from build123d import *

# Parameters (mm, degrees)
SKETCH002_R      = 1.8
SKETCH002_W      = 81
SKETCH002_H      = 81
PAD_DEPTH        = 2
SKETCH003_R      = 3.2
POCKET_DEPTH     = 0.8
SKETCH006_R      = 1.8
PAD002_DEPTH     = 0.12
PAD001_DEPTH     = 20
CHAMFER001_SIZE2 = 2.99
CHAMFER001_SIZE  = 7.5
CHAMFER002_SIZE  = 4
FILLET_R         = 4
CHAMFER003_SIZE  = 1
SKETCH005_R      = 2.2
POCKET001_DEPTH  = 33.501
SKETCH010_R      = 2.2
PAD006_DEPTH     = 0.12
SKETCH007_W      = 85
SKETCH007_H      = 85
SKETCH007_W_2    = 81
SKETCH007_H_2    = 81
PAD003_DEPTH     = 7
SKETCH008_W      = 81
SKETCH008_H      = 81
SKETCH008_R      = 2.5
PAD004_DEPTH     = 1.8
CHAMFER_SIZE     = 1.2
SKETCH009_R      = 2.5
PAD005_DEPTH     = 0.12
FILLET001_R      = 2


with BuildPart() as part:
    # Sketch002 → Pad (new body)
    with BuildSketch(Plane.XY):
        with BuildLine():
            Line((-65, 88.5), (-65, 80))
            Line((-65, 80), (-52.5, 67.5))
            Line((-52.5, 67.5), (-52.5, -20))
            Line((-52.5, -20), (-73, -20))
            Line((-73, -20), (-73, -40))
            Line((-73, -40), (-52.5, -40))
            Line((-52.5, -40), (-52.5, -50))
            Line((-52.5, -50), (52.5, -50))
            Line((52.5, -50), (52.5, -40))
            Line((52.5, -40), (91, -40))
            Line((91, -40), (91, -20))
            Line((91, -20), (52.5, -20))
            Line((52.5, -20), (52.5, 67.5))
            Line((52.5, 67.5), (120, 67.5))
            Line((120, 67.5), (133, 80.5))
            Line((133, 80.5), (133, 88.5))
            ThreePointArc((133, 88.5), (131.535534, 92.035534), (128, 93.5))
            Line((128, 93.5), (52.5, 93.5))
            ThreePointArc((52.5, 93.5), (34.115224, 85.884776), (26.5, 67.5))
            Line((26.5, 50), (26.5, 67.5))
            Line((-26.5, 50), (26.5, 50))
            Line((-26.5, 67.5), (-26.5, 50))
            ThreePointArc((-26.5, 67.5), (-34.115224, 85.884776), (-52.5, 93.5))
            Line((-60, 93.5), (-52.5, 93.5))
            ThreePointArc((-60, 93.5), (-63.535534, 92.035534), (-65, 88.5))
        make_face()
        with Locations((-60, 88.5)):
            Circle(SKETCH002_R, mode=Mode.SUBTRACT)
        with Locations((128, 85.5)):
            Circle(SKETCH002_R, mode=Mode.SUBTRACT)
        Rectangle(SKETCH002_W, SKETCH002_H, mode=Mode.SUBTRACT)
    extrude(amount=PAD_DEPTH)

    # Sketch003 → Pocket (cut)
    with BuildSketch(Plane.XY.offset(2)):
        with Locations((-60, 88.5)):
            Circle(SKETCH003_R)
        with Locations((128, 85.5)):
            Circle(SKETCH003_R)
    extrude(amount=-POCKET_DEPTH, mode=Mode.SUBTRACT)

    # Sketch006 → Pad002 (join)
    with BuildSketch(Plane.XY.offset(1.2)):
        with Locations((-60, 88.5)):
            Circle(SKETCH006_R)
        with Locations((128, 85.5)):
            Circle(SKETCH006_R)
    extrude(amount=-PAD002_DEPTH)

    # Sketch004 (on DatumPlane) → Pad001 (join)
    with BuildSketch(Plane(origin=(-87, -40, 0), x_dir=(-1, 0, 0), z_dir=(0, 1, 0))):
        Polygon((-178, 0), (-139.5, 0), (-139.5, -3), (-173, -3), (-173, -33.5), (-192, -33.5), (-192, -28.5), (-178, -28.5), align=None)
        Polygon((-14, 0), (-34.5, 0), (-34.5, -3), (-19, -3), (-19, -33.5), (0, -33.5), (0, -28.5), (-14, -28.5), align=None)
    extrude(amount=PAD001_DEPTH)

    # Chamfer001
    chamfer001_edges = [part.edges().sort_by_distance(p)[0] for p in [
        (-52.5, -30, 0),
        (52.5, -30, 0),
    ]]
    chamfer001_side = part.faces().sort_by_distance((-56.25, 91.054673, 0))[0]
    chamfer(chamfer001_edges, length=CHAMFER001_SIZE, length2=CHAMFER001_SIZE2, reference=chamfer001_side)

    # Chamfer002
    chamfer002_edges = [part.edges().sort_by_distance(p)[0] for p in [
        (91, -30, 2),
        (-73, -30, 2),
    ]]
    chamfer(chamfer002_edges, length=CHAMFER002_SIZE)

    # Fillet
    fillet_edges = [part.edges().sort_by_distance(p)[0] for p in [
        (105, -40, -31),
        (-87, -40, -31),
        (-68, -30, -33.5),
        (86, -30, -33.5),
        (-87, -20, -31),
        (105, -20, -31),
        (86, -30, -3),
        (-68, -30, -3),
        (52.5, -20, 1),
        (52.5, -40, 1),
        (52.5, -50, 1),
        (-52.5, -50, 1),
        (-52.5, -40, 1),
        (-26.5, 50, 1),
        (26.5, 50, 1),
        (52.5, 67.5, 1),
        (120, 67.5, 1),
        (133, 80.5, 1),
        (-52.5, 67.5, 1),
        (-65, 80, 1),
        (-52.5, -20, 1),
    ]]
    fillet(fillet_edges, radius=FILLET_R)

    # Chamfer003
    chamfer003_edges = [part.edges().sort_by_distance(p)[0] for p in [
        (0, 50, 2),
        (0, -50, 2),
        (91, -40, -15.25),
        (89, -40, 0),
        (89, -20, 0),
        (91, -20, -15.25),
        (-71, -40, 0),
        (-71, -20, 0),
        (-73, -20, -15.25),
        (-73, -40, -15.25),
    ]]
    chamfer(chamfer003_edges, length=CHAMFER003_SIZE)

    # Sketch005 → Pocket001 (cut, through all)
    with BuildSketch(Plane.XY):
        with Locations((-80, -30)):
            Circle(SKETCH005_R)
        with Locations((98, -30)):
            Circle(SKETCH005_R)
    extrude(amount=-POCKET001_DEPTH, mode=Mode.SUBTRACT)

    # Sketch010 (on Face105 of Pocket001) → Pad006 (join)
    with BuildSketch(Plane.XY.offset(-28.5)):
        with Locations((-80, -30)):
            Circle(SKETCH010_R)
        with Locations((98, -30)):
            Circle(SKETCH010_R)
    extrude(amount=-PAD006_DEPTH)

    # Sketch007 → Pad003 (join)
    with BuildSketch(Plane.XY):
        Rectangle(SKETCH007_W, SKETCH007_H)
        Rectangle(SKETCH007_W_2, SKETCH007_H_2, mode=Mode.SUBTRACT)
    extrude(amount=-PAD003_DEPTH)

    # Sketch008 → Pad004 (join)
    with BuildSketch(Plane.XY.offset(-7)):
        Rectangle(SKETCH008_W, SKETCH008_H)
        with Locations((-35.7, 35.7)):
            Circle(SKETCH008_R, mode=Mode.SUBTRACT)
        with Locations((35.7, 35.7)):
            Circle(SKETCH008_R, mode=Mode.SUBTRACT)
        with Locations((35.7, -35.7)):
            Circle(SKETCH008_R, mode=Mode.SUBTRACT)
        with Locations((-35.7, -35.7)):
            Circle(SKETCH008_R, mode=Mode.SUBTRACT)
    extrude(amount=PAD004_DEPTH)

    # Chamfer
    chamfer_edges = [part.edges().sort_by_distance(p)[0] for p in [
        (33.2, 35.7, -7),
        (-38.2, 35.7, -7),
        (-38.2, -35.7, -7),
        (33.2, -35.7, -7),
    ]]
    chamfer(chamfer_edges, length=CHAMFER_SIZE)

    # Sketch009 → Pad005 (join)
    with BuildSketch(Plane.XY.offset(-5.2)):
        with Locations((-35.7, 35.7)):
            Circle(SKETCH009_R)
        with Locations((35.7, 35.7)):
            Circle(SKETCH009_R)
        with Locations((35.7, -35.7)):
            Circle(SKETCH009_R)
        with Locations((-35.7, -35.7)):
            Circle(SKETCH009_R)
    extrude(amount=-PAD005_DEPTH)

    # Fillet001
    fillet001_edges = [part.edges().sort_by_distance(p)[0] for p in [
        (42.5, 42.5, -3.5),
        (-42.5, 42.5, -3.5),
        (0, 42.5, 0),
        (0, 42.5, -7),
        (-42.5, -42.5, -3.5),
        (-42.5, 0, 0),
        (-42.5, 0, -7),
        (42.5, -42.5, -3.5),
        (0, -42.5, 0),
        (0, -42.5, -7),
        (42.5, 0, 0),
        (42.5, 0, -7),
    ]]
    fillet(fillet001_edges, radius=FILLET001_R)

    # Sketch016 → Groove (revolve, cut)
    with BuildSketch(Plane.XZ):
        Polygon((0, -7), (-40.5, -7), (-41.25519, -6.1), (-40.5, -5.2), (0, -5.2), align=None)
    revolve(axis=Axis((0, 0, 0), (0, 0, 1)), mode=Mode.SUBTRACT)


solid = part.part
The model under review builds one solid part; all positions refer to its coordinate system, in mm. A direction names the side the tool comes from. Round coordinates to 2 decimals unless told otherwise and drop trailing zeros. Loops run counter-clockwise (first coordinate to the right, second up) from the corner with the lowest first, then second, coordinate; pieces in that order, holes last. Notation, with made-up numbers: M -8.5,88 L 4.5,88 A12 ccw 4.5,102 Z; hole C 53.5,68 d11. An arc over 180 degrees is marked long. Answer as CSV lines item,"result".
1. For faces 4 (the face through (-53.504, -19.063, 1.285)), 5 (the face through (97.523, -32.148, -31.026)), 6 (the face through (53.504, 66.563, 1.285)), 7 (the face through (25.297, 51.141, 0.507)), list the 3-axis set-ups (+Z, -Z, +X, -X, +Y, -Y) from which the entire face can be reached by the end or side of a thin tool; tool diameter is ignored.
Outcome:
face 4,"+Z, -X"
face 5,"-Z"
face 6,"+Z, +X"
face 7,"+Z, -Z, +Y"
2. To check wall thickness, follow L1, parallel to X at y = -1, z = -2.5; L2, parallel to Y at x = 35.7, z = -5.65; L3, parallel to Y at x = -35.7, z = -5.5. State the ranges of each line that lie inside material, in increasing order. Write a range as [from, to].
Outcome:
L1,"x = [-42.5, -40.5], [40.5, 42.5]"
L2,"y = [-42.39, -38.2], [-33.2, -19.91], [19.91, 33.2], [38.2, 42.39]"
L3,"y = [-42.44, -38.2], [-33.2, -19.65], [19.65, 33.2], [38.2, 42.44]"
3. Draft analysis for pull direction Y (two halves, no side actions). For faces 1 (the face through (-87, -30, -31)), 2 (the face through (53.703, -18.859, 0.507)), 3 (the face through (-53.703, -41.141, 0.507)), state which applies: pulls with the +Y half, pulls with the -Y half, needs draft (parallel to the pull), parting line crosses it, or undercut.
Outcome:
face 1,"needs draft"
face 2,"undercut"
face 3,"pulls with the -Y half"
4. We need section B-B (z = -13.5). Give the boundary of the cut face in (x, y), plus the area to 3 significant figures.
Outcome:
outline,"M -73,-39 L -72,-40 L -68,-40 L -68,-20 L -72,-20 L -73,-21 Z; M 86,-40 L 90,-40 L 91,-39 L 91,-21 L 90,-20 L 86,-20 Z"
area,"198 mm2"
5. Insertion check: pin 1 Ø12 at (x, z) = (-21, -12) entering from +Y; pin 2 Ø1.5 at (x, z) = (1.5, -4) entering from -Y; pin 3 Ø1 at (y, z) = (-35, -9.5) entering from -X; pin 4 Ø17 at (x, z) = (73, -12.5) entering from +Y. Each pin has a flat end and moves straight along its axis. Give the tip position at first contact, or say it passes through.
Outcome:
pin 1,"stops at y = 42.23"
pin 2,"stops at y = -42.5"
pin 3,"stops at x = -73"
pin 4,"passes through"
6. We need section A-A (y = 58.5). Give the boundary of the cut face in (x, z).
Outcome:
outline,"M -52.5,0 L -26.5,0 L -26.5,1 L -27.5,2 L -51.5,2 L -52.5,1 Z; M 26.5,0 L 52.5,0 L 52.5,1 L 51.5,2 L 27.5,2 L 26.5,1 Z"
